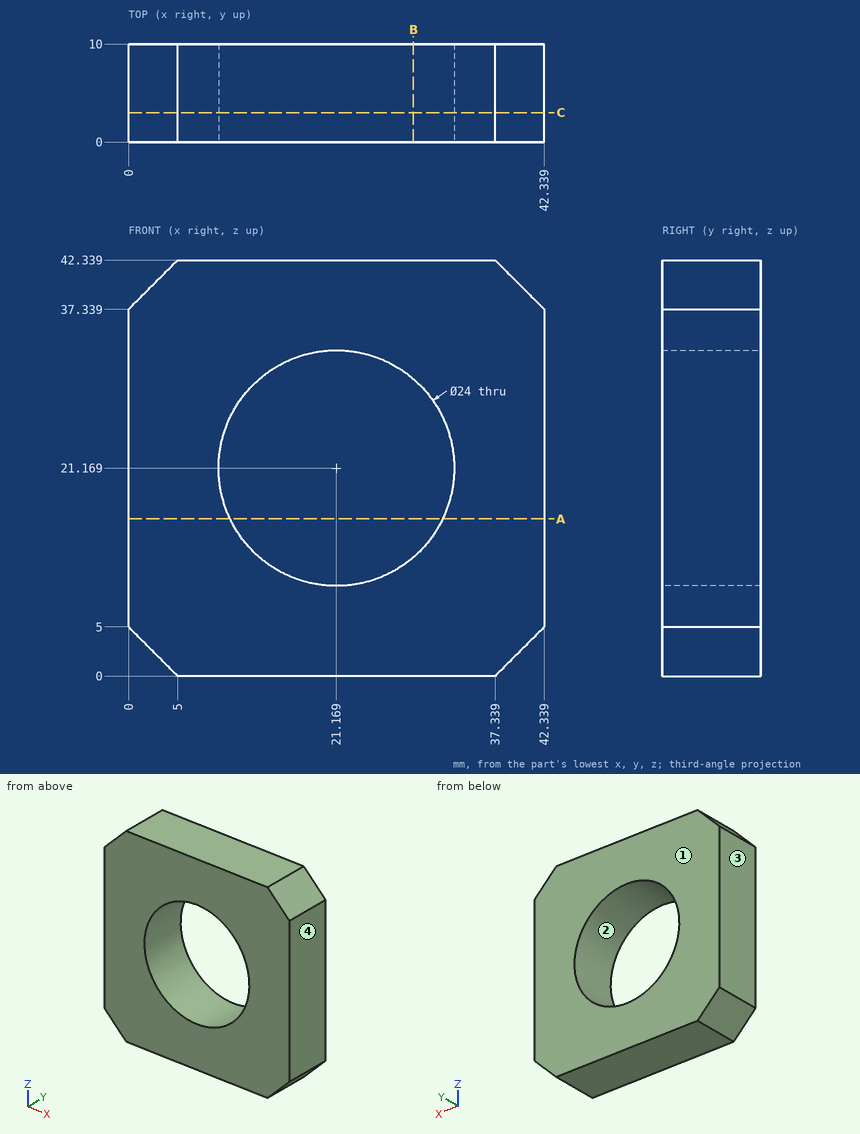
Answer from the drawing. Dimensions are ordinates in mm from the lowest x, y and z of the part. Coordinates: 2 decimals unless noted, no trailing zeros. Loops run counter-clockwise (first coordinate to the right, second up) from the corner with the lowest first, then second, coordinate; pieces in that order, holes last. Notation, with made-up numbers: (73.5, -4) -> (90.5, -4) arc R31 ccw to (90.5, 28) -> close; hole circle Ø2 at (-12.75, 58). An arc over 180 degrees is marked (long way). Return JSON: item names as keys, results as strings.
Item 1: Flat-ended cylindrical pins translate along their axes: P1, Ø5, axis at y = 2, z = 31, coming from the -X side; P2, Ø14.5, axis at x = 21.17, z = 21.17, coming from the -Y side. Find the tip coordinate at first contact, or state that the pin passes through.
Answers:
{"P1": "stops at x = 0", "P2": "passes through"}
Item 2: Find the intervals of material crossed by probe 1 along X at (y, z) = (1.75, 26) (1 decimal); probe 2 along Z at (x, y) = (17.5, 3.5) (1 decimal); probe 3 along X at (y, z) = (6.5, 23.5), in increasing order.
Answers:
{"probe 1": "x = 0 to 10.2, 32.2 to 42.3", "probe 2": "z = 0 to 9.7, 32.6 to 42.3", "probe 3": "x = 0 to 9.4, 32.94 to 42.34"}
Item 3: Find section A-A (z = 16). Determine the outline of the cut face in (x, y), plus the area to 3 significant figures.
Answers:
{"outline": "(0, 0) -> (10.34, 0) -> (10.34, 10) -> (0, 10) -> close; (32, 0) -> (42.34, 0) -> (42.34, 10) -> (32, 10) -> close", "area": "207 mm2"}
Item 4: Find section B-B (x = 29). Determine the outline of the cut face in (y, z).
Answers:
{"outline": "(0, 0) -> (10, 0) -> (10, 12.08) -> (0, 12.08) -> close; (0, 30.26) -> (10, 30.26) -> (10, 42.34) -> (0, 42.34) -> close"}
Item 5: For a pull along X with two mould halves and no side action, classify the marked faces 1, 2, 3 and 4 as +X half, -X half, draft (parallel to the pull), parting line (faces both ways), or undercut.
Answers:
{"face 1": "draft", "face 2": "undercut", "face 3": "-X half", "face 4": "+X half"}
Item 6: Find section C-C (y = 3). Determine the outline of the cut face in (x, z), plus the area to 3 significant figures.
Answers:
{"outline": "(0, 5) -> (5, 0) -> (37.34, 0) -> (42.34, 5) -> (42.34, 37.34) -> (37.34, 42.34) -> (5, 42.34) -> (0, 37.34) -> close; hole circle Ø24 at (21.17, 21.17)", "area": "1,290 mm2"}
